from build123d import *

# Parameters (mm, degrees)
BOSS_EXTRUDE1_DEPTH = 5.08
SKETCH2_W           = 12.7
SKETCH2_H           = 5.08
BOSS_EXTRUDE2_DEPTH = 6.35
FILLET3_SIZE        = 6.35
FILLET3_SIZE_2      = 12.7
FILLET4_SIZE        = 6.35
FILLET4_SIZE_2      = 12.7


with BuildPart() as part:
    # Sketch1 → Boss-Extrude1 (new body)
    with BuildSketch(Plane(origin=(0, 0, 0), x_dir=(1, 0, 0), z_dir=(0, 1, 0))):
        with BuildLine():
            Line((0, 120.65), (12.7, 120.65))
            ThreePointArc((12.7, 120.65), (89.032177029, 89.032177029), (120.65, 12.7))
            Line((120.65, 12.7), (120.65, 0))
            Line((120.65, 0), (107.95, 0))
            Line((107.95, 0), (107.95, 25.4))
            Line((107.95, 25.4), (25.4, 107.95))
            Line((25.4, 107.95), (0, 107.95))
            Line((0, 107.95), (0, 120.65))
        make_face()
        with BuildLine():
            Line((73.363460454, 75.909044866), (79.798132163, 82.343716575))
            ThreePointArc((79.798132163, 82.343716575), (82.343716575, 82.343716575), (82.343716575, 79.798132163))
            Line((82.343716575, 79.798132163), (75.909044866, 73.363460454))
            ThreePointArc((75.909044866, 73.363460454), (73.363460454, 73.363460454), (73.363460454, 75.909044866))
        make_face(mode=Mode.SUBTRACT)
    extrude(amount=BOSS_EXTRUDE1_DEPTH)

    # Sketch2 → Boss-Extrude2 (add)
    with BuildSketch(Plane.ZY):
        with Locations((-114.3, 2.54)):
            Rectangle(SKETCH2_W, SKETCH2_H)
    boss_extrude2 = extrude(amount=BOSS_EXTRUDE2_DEPTH)

    # Mirror2: Boss-Extrude2 across plane
    add(boss_extrude2.mirror(Plane(origin=(0, 0, 0), x_dir=(-0.7071067811865479, 0, 0.7071067811865471), z_dir=(0.7071067811865471, 0, 0.7071067811865479))))

    # Fillet3
    # an asymmetric fillet: 12.7, 6.35 mm, written as the material it takes off along each edge
    with BuildSketch(Plane(origin=(-6.35, 36.83, -120.65), x_dir=(1, 0, 0), z_dir=(0, -1, 0))) as fillet3_piece_1:
        with BuildLine():
            Bezier((FILLET3_SIZE, 0), (0, 0), (0, FILLET3_SIZE_2), weights=[1, 0.707106781, 1])
            Line((0, FILLET3_SIZE_2), (0, 0))
            Line((0, 0), (FILLET3_SIZE, 0))
        make_face()
    extrude(amount=68.58, mode=Mode.SUBTRACT)

    # Fillet4
    # an asymmetric fillet: 12.7, 6.35 mm, written as the material it takes off along each edge
    with BuildSketch(Plane(origin=(120.65, 36.83, 6.35), x_dir=(0, 0, -1), z_dir=(0, -1, 0))) as fillet4_piece_1:
        with BuildLine():
            Bezier((FILLET4_SIZE, 0), (0, 0), (0, -FILLET4_SIZE_2), weights=[1, 0.707106781, 1])
            Line((0, -FILLET4_SIZE_2), (0, 0))
            Line((0, 0), (FILLET4_SIZE, 0))
        make_face()
    extrude(amount=68.58, mode=Mode.SUBTRACT)


solid = part.part
Geometry: final body of the model. Coordinates: model frame, mm. A direction names the side the tool comes from. Give positions to 0.01 mm unless a question says otherwise; leave off trailing zeros. Loops run counter-clockwise (first coordinate to the right, second up) from the corner with the lowest first, then second, coordinate; pieces in that order, holes last. Notation, with made-up numbers: (28, -21) - (80, -21) arc R21 cw to (80, 12) - close; hole circle Ø2 at (81.5, -2.5). An arc over 180 degrees is marked (long way). One line per question, with ' | ' between items. Start each with the question number.
(1) Contact query for flat-ended pins moving along their axis: pin 1 (1 mm diameter, centred on x = 73.5, y = 3.5, fed in from +Z); pin 2 (1 mm diameter, centred on y = 1, z = -62.5, fed in from -X); pin 3 (2 mm diameter, centred on x = 73.5, y = 4, fed in from +Z). Output: stop coordinate, or through.
(2) Section query B-B on z = -44. Return loops of the section in (x, y).
(3) Reachability of faces 4 (the flat face through (107.95, 3, -10)), 5 (the flat face through (72, 5.08, -72)), 6 (the flat face through (76.536, 2.504, -79.081)) from +Z, -Z, +X, -X, +Y, -Y: full face, straight path, thin tool, end or side. Return the list, or none.
(4) Pull-direction query (Z, two-part tool) for faces 1 (the cylindrical face through (73.39, 2.5, -73.34)), 2 (the flat face through (120.65, 3, -6)), 3 (the flat face through (6, 3, -120.65)); classes: released by +Z, released by -Z, zero draft, split by the parting line, or undercut.
(5) Section query A-A on x = 10.5. Return loops of the section in (y, z).
(6) Ray query, line 1 (Z direction, x = 73, y = 2.3); line 2 (Z direction, x = 10, y = 0.6); line 3 (X direction, y = 0.5, z = -13). Return the intervals inside material, ascending. Write a range as from..to.
The answers:
1) pin 1: z = -59.35 | pin 2: x = 70.35 | pin 3: z = -58.85
2) outline: (89.35, 0) - (116.01, 0) - (116.01, 5.08) - (89.35, 5.08) - close
3) face 4: +Z, -X, +Y, -Y | face 5: +Z, -Z, +X, -X, +Y | face 6: +Y, -Y
4) face 1: undercut | face 2: zero draft | face 3: released by -Z
5) outline: (0, -120.65) - (5.08, -120.65) - (5.08, -107.95) - (0, -107.95) - close
6) line 1: -102.24..-75.39, -73.89..-60.35 | line 2: -120.65..-107.95 | line 3: 107.95..120.65
